Design review of the part built by this model. Coordinates are the model's own, in mm. Face numbers are marked on the shaded views. A direction names the side the tool comes from. Coordinates: 2 decimals unless noted, no trailing zeros. Loops run counter-clockwise (first coordinate to the right, second up) from the corner with the lowest first, then second, coordinate; pieces in that order, holes last. Notation, with made-up numbers: (78.5, -34.5) - (87.5, -34.5) arc R18 ccw to (87.5, -6.5) - close; hole circle Ø7 at (-2.75, 43). An arc over 180 degrees is marked (long way). Use one line per item in the form item = value. Start each with the question number.
(1) Add section C-C (x = 22.5). State the section outline as (y, z) points.
(2) Tool access review of the marked faces 1, 2, 3 and 4: name each direction out of +Z, -Z, +X, -X, +Y, -Y from which nothing blocks a thin tool from reaching the whole face with its end or side.
(3) Add section B-B (z = 0). State the section outline as (x, y) points.
(4) Add section A-A (y = -11.5). State the section outline as (x, z) points, plus the area to 3 significant figures.
(5) The part is to be moulded in two halves that separate along X. For the marked faces 5, 6, 7 and 8, say which applies: pulls with the +X half, pulls with the -X half, needs draft (parallel to the pull), parting line crosses it, or undercut.
(6) Clearance check with flat-ended pins moving along their axes: pin 1 Ø19 at (x, z) = (-12, -21) entering from +Y; pin 2 Ø6.5 at (x, z) = (28.5, -13.5) entering from -Y; pin 3 Ø2 at (y, z) = (-2, -3) entering from +X; pin 4 Ø6.5 at (x, z) = (-25.5, 11.5) entering from -Y. State where each tip first meets the part, or that it passes through.
(7) For L1, parallel to Z at x = -35, y = -11.5; L2, parallel to X at y = -11.75, z = 22; L3, parallel to X at y = 4, z = 1, list the stretches that pass through material, from the lowest coordinate up.
(8) Add section D-D (x = -53.5). State the section outline as (y, z) points.
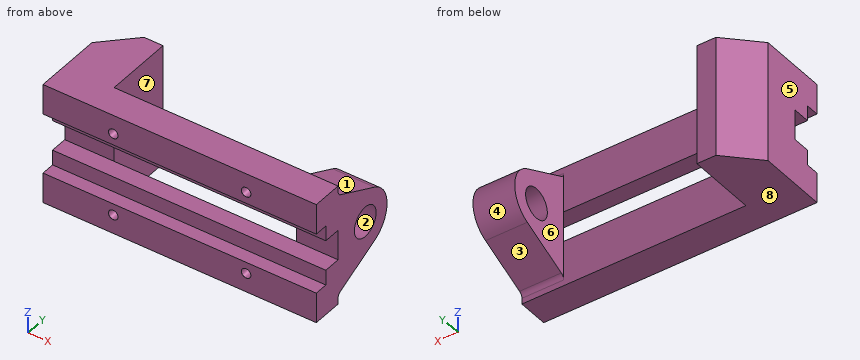
```python
from build123d import *

# Parameters (mm, degrees)
SKETCH1_W                             = 144
SKETCH1_H                             = 64
BOSS_EXTRUDE1_DEPTH                   = 16
CUT_EXTRUDE1_REACH                    = 146
BOSS_EXTRUDE2_DEPTH                   = 32
SKETCH5_R                             = 8
BOSS_EXTRUDE3_DEPTH                   = 22
FILLET1_R                             = 3
TAP_DRILL_FOR_M6X1_0_TAP1_D           = 5
TAP_DRILL_FOR_M6X1_0_TAP1_DEPTH       = 8.497848452
TAP_DRILL_FOR_M6X1_0_TAP1_CSINK_D     = 5.05
TAP_DRILL_FOR_M6X1_0_TAP1_CSINK_ANGLE = 90
TAP_DRILL_FOR_M6X1_0_TAP1_TIP         = 1.502151548


with BuildPart() as part:
    # Sketch1 → Boss-Extrude1 (new body)
    with BuildSketch(Plane(origin=(0, 0, 0), x_dir=(1, 0, 0), z_dir=(0, 1, 0))):
        Rectangle(SKETCH1_W, SKETCH1_H)
    extrude(amount=-BOSS_EXTRUDE1_DEPTH)

    # Sketch2 → Cut-Extrude1 (cut, up to next)
    with BuildSketch(Plane(origin=(72, 0, 0), x_dir=(0, 0, -1), z_dir=(1, 0, 0)), mode=Mode.PRIVATE) as cut_extrude1_sk1:
        Polygon((-8, 0), (8, 0), (8, -9), (16, -9), (16, -16), (-16, -16), (-16, -9), (-8, -9), align=None)
    cut_extrude1_tool1 = extrude(cut_extrude1_sk1.sketch, amount=-CUT_EXTRUDE1_REACH, mode=Mode.PRIVATE) & part.part
    add(cut_extrude1_tool1.solids().sort_by_distance((72, -9.369565, 0))[0], mode=Mode.SUBTRACT)

    # Sketch4 → Boss-Extrude2 (add, symmetric)
    with BuildSketch(Plane.XY):
        Polygon((-72, 20), (-56, 36), (-46, 36), (-46, 0), (-72, 0), align=None)
    extrude(amount=BOSS_EXTRUDE2_DEPTH, both=True)

    # Sketch5 → Boss-Extrude3 (add)
    with BuildSketch(Plane(origin=(72, 0, 0), x_dir=(0, 0, -1), z_dir=(1, 0, 0))):
        with BuildLine():
            Line((26.980199866, 0), (14.500924593, 26.761892188))
            ThreePointArc((14.500924593, 26.761892188), (0, 36), (-14.500924593, 26.761892188))
            Line((-14.500924593, 26.761892188), (-26.980199866, 0))
            Line((-26.980199866, 0), (26.980199866, 0))
        make_face()
        with Locations((0, 20)):
            Circle(SKETCH5_R, mode=Mode.SUBTRACT)
    extrude(amount=-BOSS_EXTRUDE3_DEPTH)

    # Fillet1
    fillet1_edges = [part.edges().sort_by_distance(p)[0] for p in [
        (61, 0, -26.980199866),
        (61, 0, 26.980199866),
    ]]
    fillet(fillet1_edges, radius=FILLET1_R)

    # Tap Drill for M6x1.0 Tap1
    with Locations(Plane(origin=(0, -16, 0), x_dir=(-1, 0, 0), z_dir=(0, -1, 0))):
        with Locations((35, 22), (-35, 22), (35, -22), (-35, -22), (0, 0)):
            CounterSinkHole(TAP_DRILL_FOR_M6X1_0_TAP1_D / 2, TAP_DRILL_FOR_M6X1_0_TAP1_CSINK_D / 2, depth=TAP_DRILL_FOR_M6X1_0_TAP1_DEPTH, counter_sink_angle=TAP_DRILL_FOR_M6X1_0_TAP1_CSINK_ANGLE)
            with Locations((0, 0, -(TAP_DRILL_FOR_M6X1_0_TAP1_DEPTH + TAP_DRILL_FOR_M6X1_0_TAP1_TIP / 2))):  # 118° drill point
                Cone(0, TAP_DRILL_FOR_M6X1_0_TAP1_D / 2, TAP_DRILL_FOR_M6X1_0_TAP1_TIP, mode=Mode.SUBTRACT)


solid = part.part
```
Computed values:
q1.outline = (-16, -32) - (0, -32) - (0, -8) - (-9, -8) - (-9, -16) - (-16, -16) - close; (-16, 16) - (-9, 16) - (-9, 8) - (0, 8) - (0, 32) - (-16, 32) - close
q2.face_1 = +Z, +X, +Y
q2.face_2 = +X
q2.face_3 = -Z, +X, +Y
q2.face_4 = +X, +Y
q3.outline = (-72, 0) - (-46, 0) - (-46, 36) - (-56, 36) - (-72, 20) - close; (50, 0) - (72, 0) - (72, 12) - (50, 12) - close; (50, 28) - (72, 28) - (72, 36) - (50, 36) - close
q4.outline = (-72, -32) - (72, -32) - (72, -16) - (-72, -16) - close; (-72, 16) - (72, 16) - (72, 32) - (-72, 32) - close; hole circle Ø5 at (-35, -22); hole circle Ø5 at (-35, 22); hole circle Ø5 at (35, -22); hole circle Ø5 at (35, 22)
q4.area = 4,530 mm^2
q5.face_5 = pulls with the -X half
q5.face_6 = undercut
q5.face_7 = undercut
q5.face_8 = needs draft
q6.pin_1 = 0
q6.pin_2 = -16
q6.pin_3 = through
q6.pin_4 = -9
q7.L1 = -32 to -24.5, -19.5 to -16, 16 to 19.5, 24.5 to 32
q7.L2 = -72 to -37.5, -32.5 to 32.5, 37.5 to 72
q7.L3 = -72 to -46, 50 to 72
q8.outline = (-16, -32) - (36, -32) - (36, 32) - (-16, 32) - (-16, 16) - (-9, 16) - (-9, 8) - (0, 8) - (0, -8) - (-9, -8) - (-9, -16) - (-16, -16) - close
